CAD build for the part. Positions are in the model's coordinates, mm. Face numbers are marked on the shaded views. A direction names the side the tool comes from. Coordinates: 2 decimals unless noted, no trailing zeros. Order: outer loops, then holes, each group sorted by start corner. A loop starts at its lowest first (then second) coordinate and runs counter-clockwise, first axis right, second up. Notation, with made-up numbers: (50, 5) - (80, 5) arc R30 ccw to (80, 40) - close; hole circle Ø9 at (-17, 22.25). An arc over 180 degrees is marked (long way). Use one line per item in the form item = value.
Autodesk Inventor part; units mm, degrees
ref_plane "YZ Plane" through (0, 0, 0) normal (1, 0, 0) x (0, 1, 0)
ref_plane "XZ Plane" through (0, 0, 0) normal (0, 1, 0) x (-1, 0, 0)
ref_plane "XY Plane" through (0, 0, 0) normal (0, 0, 1) x (1, 0, 0)
ref_plane "작업 평면1" through (0, 0, 0) normal (0, 0, 1) x (1, 0, 0)
sketch "스케치1" plane through (0, 0, 0) normal (0, 0, 1) x (1, 0, 0)
  line L0 (12.7, -89.2) -> (9.2, -89.2)
  line L1 (12.7, -89.2) -> (17.8, -83.2)
  line L2 (17.8, -83.2) -> (17.8, -44.6)
  line L3 (17.8, -44.6) -> (12.7, -38.6)
  line L4 (12.7, -38.6) -> (-12.7, -38.6)
  line L5 (-12.7, -38.6) -> (-17.8, -44.6)
  line L6 (-17.8, -44.6) -> (-17.8, -83.2)
  line L7 (-17.8, -83.2) -> (-12.7, -89.2)
  line L8 (-9.2, -89.2) -> (-12.7, -89.2)
  arc A0 (-12.2, -86.2) -> (-9.2, -89.2) centre (-9.2, -86.2) ccw
  line L9 (-12.2, -47.2) -> (-12.2, -86.2)
  arc A1 (-9.2, -44.2) -> (-12.2, -47.2) centre (-9.2, -47.2) ccw
  line L10 (9.2, -44.2) -> (-9.2, -44.2)
  arc A2 (12.2, -47.2) -> (9.2, -44.2) centre (9.2, -47.2) ccw
  line L11 (12.2, -86.2) -> (12.2, -47.2)
  arc A3 (9.2, -89.2) -> (12.2, -86.2) centre (9.2, -86.2) ccw
  circle A4 centre (15, -81.7) radius 1.35
  circle A5 centre (15, -64.7) radius 1.35
  circle A6 centre (8.5, -41.4) radius 1.35
  circle A7 centre (-15, -81.7) radius 1.35
  circle A8 centre (-15, -64.7) radius 1.35
  circle A9 centre (-8.5, -41.4) radius 1.35
  circle A10 centre (15, -47.7) radius 1.35
  circle A11 centre (-15, -47.7) radius 1.35
  line L12 (-12.7, 12) -> (-9.2, 12)
  line L13 (-12.7, 12) -> (-17.8, 6)
  line L14 (-17.8, 6) -> (-17.8, -32.6)
  line L15 (-17.8, -32.6) -> (-12.7, -38.6)
  line L16 (-12.7, -38.6) -> (12.7, -38.6)
  line L17 (12.7, -38.6) -> (17.8, -32.6)
  line L18 (17.8, -32.6) -> (17.8, 6)
  line L19 (17.8, 6) -> (12.7, 12)
  line L20 (9.2, 12) -> (12.7, 12)
  arc A12 (12.2, 9) -> (9.2, 12) centre (9.2, 9) ccw
  line L21 (12.2, -30) -> (12.2, 9)
  arc A13 (9.2, -33) -> (12.2, -30) centre (9.2, -30) ccw
  line L22 (-9.2, -33) -> (9.2, -33)
  arc A14 (-12.2, -30) -> (-9.2, -33) centre (-9.2, -30) ccw
  line L23 (-12.2, 9) -> (-12.2, -30)
  arc A15 (-9.2, 12) -> (-12.2, 9) centre (-9.2, 9) ccw
  circle A16 centre (-15, 4.5) radius 1.35
  circle A17 centre (-15, -12.5) radius 1.35
  circle A18 centre (-8.5, -35.8) radius 1.35
  circle A19 centre (15, 4.5) radius 1.35
  circle A20 centre (15, -12.5) radius 1.35
  circle A21 centre (8.5, -35.8) radius 1.35
  circle A22 centre (-15, -29.5) radius 1.35
  circle A23 centre (15, -29.5) radius 1.35
  line L24 (-8.5, -43.8367) -> (-8.5, -33.6588)
  line L25 (-8.5, -33.6588) -> (8.5, -33.6588)
  line L26 (8.5, -33.6588) -> (8.5, -43.8367)
  line L27 (8.5, -43.8367) -> (-8.5, -43.8367)
  line L28 (-8.5, -43.8367) -> (-8.5, -33.6588)
  line L29 (-8.5, -33.6588) -> (-11.5, -33.6588)
  line L30 (-11.5, -33.6588) -> (-11.5, -43.8367)
  line L31 (-11.5, -43.8367) -> (-8.5, -43.8367)
  line L32 (8.5, -43.8367) -> (8.5, -33.6588)
  line L33 (8.5, -33.6588) -> (11.5, -33.6588)
  line L34 (11.5, -33.6588) -> (11.5, -43.8367)
  line L35 (11.5, -43.8367) -> (8.5, -43.8367)
  circle A24 centre (15, -47.7) radius 2.8
  circle A25 centre (15, -29.5) radius 2.8
  circle A26 centre (-15, -47.7) radius 2.8
  circle A27 centre (-15, -29.5) radius 2.8
  line L36 (17.8, -50.175) -> (13.5711, -50.175)
  line L37 (13.5711, -27.025) -> (17.8, -27.025)
  line L38 (-13.5711, -50.175) -> (-17.8, -50.175)
  line L39 (-17.8, -27.025) -> (-13.5711, -27.025)
  circle A28 centre (15, -47.7) radius 2.475
  circle A29 centre (15, -29.5) radius 2.475
  circle A30 centre (-15, -47.7) radius 2.475
  circle A31 centre (-15, -29.5) radius 2.475
  line L40 (15, -29.5) -> (11.5, -29.5)
  line L41 (12.525, -29.5) -> (12.525, -47.7)
  line L42 (12.525, -47.7) -> (12.525, -49.0093)
  line L43 (12.525, -29.5) -> (12.525, -28.1907)
  circle A32 centre (9.2, -47.2) radius 4.0745
  circle A33 centre (9.2, -30) radius 4.3217
  circle A34 centre (9.2, -47.2) radius 8.2366
  circle A35 centre (9.2, -30) radius 8.2366
  circle A36 centre (-9.2, -47.2) radius 8.2366
  circle A37 centre (-9.2, -30) radius 8.2439
  circle A38 centre (-9.2, -47.2) radius 4.0745
  circle A39 centre (-9.2, -30) radius 4.3217
  point P0 (0, 0)
  point P1 (-13.3169, -31.3146)
  point P2 (-17.3396, -28.6926)
  point P3 (-15.7015, -35.0688)
  point P4 (-15.25, -35.6)
  point P5 (-11.5, -37.9166)
  point P6 (-11.5, -39.2911)
  point P7 (-17.3258, -48.5464)
  point P8 (-13.1204, -46.0899)
  point P9 (12.525, -44.845)
  point P10 (17.3258, -48.5464)
  point P11 (12.525, -39.6644)
  point P12 (12.525, -37.5356)
  point P13 (17.3258, -28.6536)
  point P14 (12.525, -32.7607)
  dimension "d0" = 3
  dimension "d1" = 3
extrude "돌출2" add sketch "스케치1" along normal blind 6 contours A34 A28 A32 A24 | A24 A32 L41 A34 | A34 L26 A6 A32 L27 | L27 A36 L24 L4 L26 A34 | A32 A28 L41 A24 | A24 L41 A32 | A28 A32 A34 | A32 L26 L27 | A28 A32 | L27 A38 L24 A9 A36 | A34 L34 A32 L26 A6 | L26 L4 L34 A34 | A34 L34 L4 L41 | L41 A32 L34 A34 | L26 A32 L35 | L27 L24 A38 | A36 L30 L4 L24 | L24 A9 A38 L30 A36 | L26 A35 L34 L4 | L4 L24 A37 L25 A35 L26 | L4 L34 A35 L41 | A35 L41 A33 A25 | L31 A38 L24 | L4 L30 A37 L24 | L30 A38 A26 A36 | A35 L25 A33 L26 A21 | L26 A21 A33 L34 A35 | A35 L34 A33 L41 | A25 A33 A29 A35 | A37 L30 A39 L24 A18 | L24 A18 A39 L25 A37 | L41 A25 A33 | A25 L41 A29 A33 | A38 A30 A36 A26 | A38 A30 | A30 A36 A38 | A37 L15 A27 A39 L30 | A33 L26 L33 | L25 L26 A33 | A33 A29 A35 | A29 L40 A33 | L29 L24 A39 | A39 L24 L25 | A29 A33 L40 | A27 A37 A31 A39 | A39 A31 | A31 A37 A39
sketch "스케치2" plane through (0, 0, 6) normal (0, 0, 1) x (1, 0, 0)
  line L0 (11.5, -33.6588) -> (-11.5, -33.6588)
  arc A0 (-13.3169, -31.3146) -> (-11.5, -33.6588) centre (-9.2, -30) ccw
  arc A1 (-13.3169, -31.3146) -> (-17.3396, -28.6926) centre (-15, -29.5) ccw
  arc A2 (-17.3396, -28.6926) -> (-15.7015, -35.0688) centre (-9.2, -30) ccw
  line L1 (-15.7015, -35.0688) -> (-15.25, -35.6)
  arc A3 (-15.25, -35.6) -> (-11.5, -37.9166) centre (-9.2, -30) ccw
  line L2 (-11.5, -37.9166) -> (-11.5, -39.2911)
  arc A4 (-11.5, -39.2911) -> (-17.3258, -48.5464) centre (-9.2, -47.2) ccw
  arc A5 (-17.3258, -48.5464) -> (-13.1204, -46.0899) centre (-15, -47.7) ccw
  arc A6 (-11.5, -43.8367) -> (-13.1204, -46.0899) centre (-9.2, -47.2) ccw
  line L3 (-11.5, -43.8367) -> (11.5, -43.8367)
  arc A7 (12.525, -44.845) -> (11.5, -43.8367) centre (9.2, -47.2) ccw
  line L4 (12.525, -44.845) -> (12.525, -47.7)
  arc A8 (12.525, -47.7) -> (17.3258, -48.5464) centre (15, -47.7) ccw
  arc A9 (17.3258, -48.5464) -> (12.525, -39.6644) centre (9.2, -47.2) ccw
  line L5 (12.525, -39.6644) -> (12.525, -37.5356)
  arc A10 (12.525, -37.5356) -> (17.3258, -28.6536) centre (9.2, -30) ccw
  arc A11 (17.3258, -28.6536) -> (12.525, -29.5) centre (15, -29.5) ccw
  line L6 (12.525, -29.5) -> (12.525, -32.7607)
  arc A12 (11.5, -33.6588) -> (12.525, -32.7607) centre (9.2, -30) ccw
  circle A13 centre (15, -47.7) radius 1.35
  circle A14 centre (8.5, -35.8) radius 1.35
  circle A15 centre (15, -29.5) radius 1.35
  circle A16 centre (8.5, -41.4) radius 1.35
  circle A17 centre (-8.5, -41.4) radius 1.35
  circle A18 centre (-15, -47.7) radius 1.35
  circle A19 centre (-15, -29.5) radius 1.35
  circle A20 centre (-8.5, -35.8) radius 1.35
  line L7 (-17.4288, -29.5) -> (17.4214, -29.5)
  line L8 (-15, -47.7) -> (17.4214, -47.7)
  line L9 (-15, -47.7) -> (-18, -47.7)
  line L10 (-15, -47.7) -> (-12, -47.7) construction
  line L11 (17.4214, -29.5) -> (17.4214, -47.7)
  line L12 (17.4214, -47.7) -> (-17.4288, -47.7)
  line L13 (-17.4288, -47.7) -> (-17.4288, -29.5)
  line L14 (-17.4288, -29.5) -> (17.4214, -29.5)
  point P0 (0, 0)
  point P1 (17.4214, -46.7)
  point P2 (17.4214, -30.5)
  point P3 (-17.4288, -30.5)
  point P4 (-17.4288, -46.8415)
  dimension "d6" = 3
  dimension "d7" = 180
extrude "돌출3" add sketch "스케치2" against normal blind 6 contours L11 A9 L5 A10 | A2 L1 A3 L2 A4 L13
properties part number "_arm_adt" material "PMMA 플라스틱"
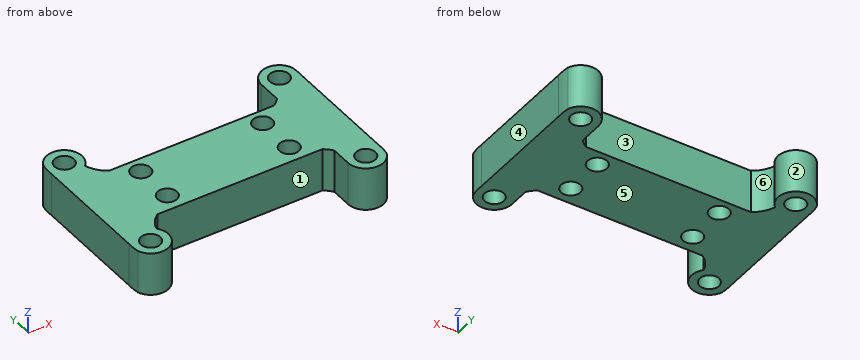
Item 1: Drop flat-ended pins along their axis: pin 1 (0.9 mm diameter, centred on y = -47, z = 3, fed in from -X); pin 2 (1.5 mm diameter, centred on y = -33, z = 3, fed in from +X); pin 3 (2 mm diameter, centred on x = 8.5, y = -35.8, fed in from -Z); pin 4 (1.5 mm diameter, centred on x = 3.5, z = 2, fed in from +Y). Give the stop position or say it passes through.
Derived:
pin_1 = -17.44
pin_2 = 17.42
pin_3 = through
pin_4 = -33.66
Item 2: Drill centre lines: line 1 (Y direction, x = -8.5, z = 0.5); line 2 (Y direction, x = 15, z = 4.45) (3 decimals); line 3 (X direction, y = -35.8, z = 2.95). Where is each one in solid material? Low to high. Write a range as [from, to].
Derived:
line_1 = [-43.84, -42.75], [-40.05, -37.15], [-34.45, -33.66]
line_2 = [-50.175, -49.05], [-46.35, -30.85], [-28.15, -27.025]
line_3 = [-17.43, -9.85], [-7.15, 7.15], [9.85, 17.42]
Item 3: Cut at A-A, the plane y = -41.4. Write the cut outline in (x, z).
Derived:
outline = (-17.43, 0) - (-9.85, 0) - (-9.85, 6) - (-17.43, 6) - close; (-7.15, 0) - (7.15, 0) - (7.15, 6) - (-7.15, 6) - close; (9.85, 0) - (17.42, 0) - (17.42, 6) - (9.85, 6) - close
Item 4: 3-axis set-ups, long thin cutter, end or side, ignore diameter. For the marked faces 1, 2 and 3: which of +Z, -Z, +X, -X, +Y, -Y reach the whole face in a straight line?
Derived:
face_1 = +Z, -Z, -Y
face_2 = +Z, -Z
face_3 = +Z, -Z, +Y
Item 5: Cut at B-B, the plane x = 15. Write the cut outline in (y, z) (3 decimals).
Derived:
outline = (-50.175, 0) - (-49.05, 0) - (-49.05, 6) - (-50.175, 6) - close; (-46.35, 0) - (-30.85, 0) - (-30.85, 6) - (-46.35, 6) - close; (-28.15, 0) - (-27.025, 0) - (-27.025, 6) - (-28.15, 6) - close
Item 6: Two-plate mould, pull along X, no slides. Class the marked faces 4, 5 and 6: +X half, -X half, draft (parallel to the pull), parting line (faces both ways), or undercut.
Derived:
face_4 = +X half
face_5 = draft
face_6 = undercut
Item 7: Cut at D-D, the plane x = 6.5. Write the cut outline in (y, z).
Derived:
outline = (-43.84, 0) - (-33.66, 0) - (-33.66, 6) - (-43.84, 6) - close
Item 8: Cut at C-C, the plane z = 5.5. State how many separate pieces and enclosed holes the cut face has, plus the area to 3 significant figures.
Derived:
separate_pieces = 1
enclosed_holes = 8
area = 426 mm²
